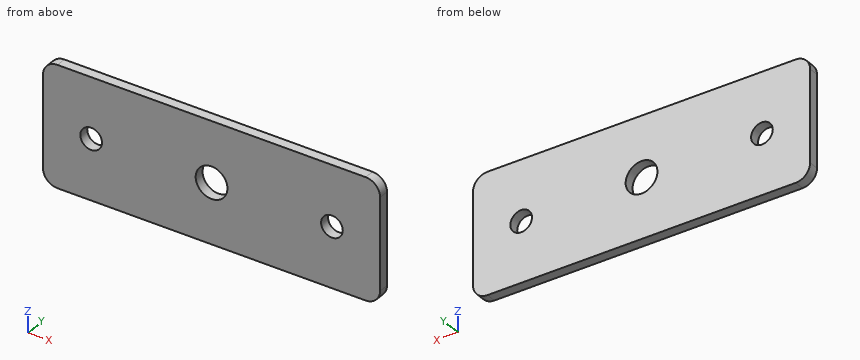
Autodesk Inventor part; units mm, degrees
ref_plane "YZ Plane" through (0, 0, 0) normal (1, 0, 0) x (0, 1, 0)
ref_plane "XZ Plane" through (0, 0, 0) normal (0, 1, 0) x (-1, 0, 0)
ref_plane "XY Plane" through (0, 0, 0) normal (0, 0, 1) x (1, 0, 0)
sketch "Sketch1" plane through (0, 0, 0) normal (0, 1, 0) x (-1, 0, 0)
  line L0 (35, -12.5) -> (-35, -12.5)
  line L1 (-35, -12.5) -> (-35, 12.5)
  line L2 (-35, 12.5) -> (35, 12.5)
  line L3 (35, 12.5) -> (35, -12.5)
  line L4 (35, -12.5) -> (-35, 12.5) construction
  line L5 (-35, -12.5) -> (35, 12.5) construction
  point P0 (0, 0)
  point P1 (0, 0)
  dimension "d19" = 25
  dimension "d21" = 70
extrude "Plate1" add sketch "Sketch1" along normal blind 2.1
sketch "Sketch2" plane through (0, 2.1, 0) normal (0, 1, 0) x (1, 0, 0)
  line L0 (0, 0) -> (-25, 0)
  line L1 (0, 0) -> (0, 5)
  point P0 (25, 0)
  point P1 (25, 0)
  dimension "d3" = 25
  dimension "d4" = 5
hole "Hole1" at (0, 2.1, 0) direction (0, -1, 0) diameter 6.6 depth 2.1
hole "Hole2" at (-25, 2.1, 0) at (25, 2.1, 0) direction (0, -1, 0) diameter 4.5 depth 2.1
fillet "Corner Round1" radius 3 4 edges at (-35, 1.05, 12.5) (35, 1.05, 12.5) (35, 1.05, -12.5) (-35, 1.05, -12.5)
equation "\"d10\" = Thickness"
equation "\"d17\" = Thickness"
equation "\"d2\" = Thickness"
equation "\"BendReliefWidth\" = Thickness"
equation "\"BendReliefDepth\" = 0.5 * Thickness"
equation "\"CornerReliefSize\" = 4 * Thickness"
equation "\"MinimumRemnant\" = 2 * Thickness"
equation "\"TransitionRadius\" = BendRadius"
equation "\"JacobiRadiusSize\" = BendRadius"
equation "\"GapSize\" = Thickness"
properties part number "SP58V1 Seguro Pedales" material "Steel, Carbon"
Here's how the part is built. I have some questions about the finished solid (model axes, mm). Give positions to 0.01 mm unless a question says otherwise; leave off trailing zeros. Loops run counter-clockwise (first coordinate to the right, second up) from the corner with the lowest first, then second, coordinate; pieces in that order, holes last. Notation, with made-up numbers: (57, 40) -> (71, 40) arc R19 cw to (71, 66) -> close; hole circle Ø6 at (-31.5, 79.5). An arc over 180 degrees is marked (long way). One line per item, written item: value.
Q1. Suppose I cut it at C-C on y = 1.4. Please give me the cut outline in (x, z).
Answers follow:
outline: (-35, -9.5) arc R3 ccw to (-32, -12.5) -> (32, -12.5) arc R3 ccw to (35, -9.5) -> (35, 9.5) arc R3 ccw to (32, 12.5) -> (-32, 12.5) arc R3 ccw to (-35, 9.5) -> close; hole circle Ø4.5 at (-25, 0); hole circle Ø6.6 at (0, 0); hole circle Ø4.5 at (25, 0)
Q2. I'm going to push a flat-ended pin straight in: pin 1 Ø4 at (x, z) = (25, 0) entering from +Y. Where does the tip first touch, or does it pass through?
Answers follow:
pin 1: through
Q3. Suppose I cut it at A-A on z = 0. Please give me the cut outline in (x, y).
Answers follow:
outline: (-35, 0) -> (-27.25, 0) -> (-27.25, 2.1) -> (-35, 2.1) -> close; (-22.75, 0) -> (-3.3, 0) -> (-3.3, 2.1) -> (-22.75, 2.1) -> close; (3.3, 0) -> (22.75, 0) -> (22.75, 2.1) -> (3.3, 2.1) -> close; (27.25, 0) -> (35, 0) -> (35, 2.1) -> (27.25, 2.1) -> close
Q4. If I drill on line 1 along X through (y, z) = (0.8, 0); line 2 along Z through (x, y) = (25, 1.5); line 3 along Z through (x, y) = (0, 1.6), over which ranges is the centre line in solid material (lowest first)?
Answers follow:
line 1: -35 to -27.25, -22.75 to -3.3, 3.3 to 22.75, 27.25 to 35
line 2: -12.5 to -2.25, 2.25 to 12.5
line 3: -12.5 to -3.3, 3.3 to 12.5
Q5. Suppose I cut it at D-D on x = 0. Please give me the cut outline in (y, z), then the cut area to 3 significant figures.
Answers follow:
outline: (0, -12.5) -> (2.1, -12.5) -> (2.1, -3.3) -> (0, -3.3) -> close; (0, 3.3) -> (2.1, 3.3) -> (2.1, 12.5) -> (0, 12.5) -> close
area: 38.6 mm^2
Q6. Suppose I cut it at B-B on x = 25. Please give me the cut outline in (y, z).
Answers follow:
outline: (0, -12.5) -> (2.1, -12.5) -> (2.1, -2.25) -> (0, -2.25) -> close; (0, 2.25) -> (2.1, 2.25) -> (2.1, 12.5) -> (0, 12.5) -> close
